Geometry: final body of the model. Coordinates: model frame, mm. Round coordinates to 2 decimals unless told otherwise and drop trailing zeros. Write each loop counter-clockwise with the first axis right and the second up, starting at its lowest first coordinate (ties: lowest second). Pieces come first, ordered by that corner, then holes. Notation, with made-up numbers: M -8,59 L 21,59 A27 cw 21,82 Z; hole C 0,-30 d11. An arc over 180 degrees is marked long. Answer as CSV lines item,"result". Start each with the question number.
Q1. Section query D-D on x = 29.5. Output: boundary loops of the cut face in (y, z) (3 decimals).
Q2. First-contact query: pin 1 (0.5 mm diameter, centred on y = -0.5, z = 0, fed in from -X); pin 2 (0.8 mm diameter, centred on y = 0, z = -15.5, fed in from -X); pin 3 (0.8 mm diameter, centred on x = 34, y = 0, fed in from +Z). Flat tips, straight axial feed; report the tip coordinate or a pass-through.
Q3. Section query B-B on x = -2.5. Output: boundary loops of the cut face in (y, z) (3 decimals).
Q4. Section query A-A on z = -2.5. Output: boundary loops of the cut face in (x, y) (3 decimals), and give its area (3 significant figures).
Q5. Ray query, probe 1 along X at (y, z) = (0.4, 4.5); probe 2 along X at (y, z) = (-0.3, 1); probe 3 along Z at (x, y) = (-8.5, 0.7). Return the intervals inside material, ascending.
Q6. Section query C-C on y = 0.3. Give the number of separate pieces and of enclosed holes in the cut face, and give its area (3 significant figures).
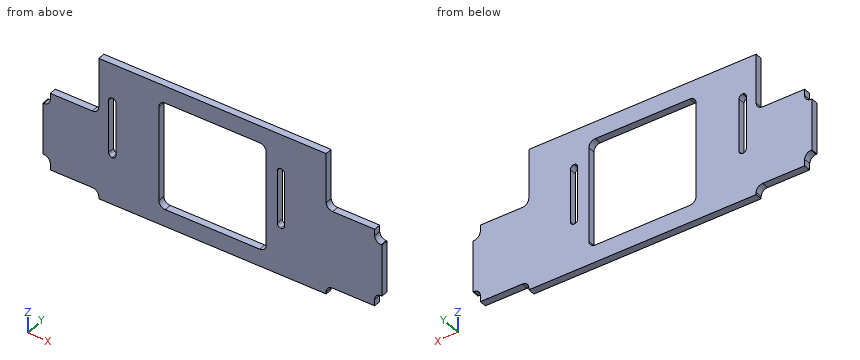
```python
from build123d import *

# Parameters (mm, degrees)
SKIZZE1_W                       = 1.7
SKIZZE1_H                       = 14
SKIZZE1_W_2                     = 25
SKIZZE1_H_2                     = 25
AUFSATZ_LINEAR_AUSTRAGEN1_DEPTH = 0.825
VERRUNDUNG1_R                   = 1.5
VERRUNDUNG2_R                   = 0.85


with BuildPart() as part:
    # Skizze1 → Aufsatz-Linear austragen1 (new, symmetric)
    # profile 1 of 3: a face of its own
    with BuildSketch(Plane(origin=(0, 0, 0), x_dir=(1, 0, 0), z_dir=(0, 1, 0))):
        Polygon((26.5, 16), (26.5, 18), (-26.5, 18), (-26.5, 16), (-26.5, -2), (-26.5, -15), (26.5, -15), (26.5, -2), align=None)
        with Locations((-23.35, 0)):
            Rectangle(SKIZZE1_W, SKIZZE1_H, mode=Mode.SUBTRACT)
        with Locations((15.95, 0)):
            Rectangle(SKIZZE1_W, SKIZZE1_H, mode=Mode.SUBTRACT)
        with Locations((0, 1.5)):
            Rectangle(SKIZZE1_W_2, SKIZZE1_H_2, mode=Mode.SUBTRACT)
    # profile 2 of 3: a face of its own
    with BuildSketch(Plane(origin=(0, 0, 0), x_dir=(1, 0, 0), z_dir=(0, 1, 0))):
        Polygon((-26.5, -2), (-26.5, 16), (-37.8, 16), (-37.8, 13), (-39.5, 13), (-39.5, 1), (-37.8, 1), (-37.8, -2), align=None)
    # profile 3 of 3: a face of its own
    with BuildSketch(Plane(origin=(0, 0, 0), x_dir=(1, 0, 0), z_dir=(0, 1, 0))):
        Polygon((37.8, 16), (26.5, 16), (26.5, -2), (37.8, -2), (37.8, 1), (39.5, 1), (39.5, 13), (37.8, 13), align=None)
    extrude(amount=AUFSATZ_LINEAR_AUSTRAGEN1_DEPTH, both=True)

    # Verrundung1
    verrundung1_edges = [part.edges().sort_by_distance(p)[0] for p in [
        (-26.5, 0, 2),
        (-37.8, 0, -1),
        (-37.8, 0, -13),
        (-26.5, 0, -16),
        (26.5, 0, -16),
        (37.8, 0, -13),
        (37.8, 0, -1),
        (26.5, 0, 2),
        (-12.5, 0, -14),
        (-12.5, 0, 11),
        (12.5, 0, 11),
        (12.5, 0, -14),
    ]]
    fillet(verrundung1_edges, radius=VERRUNDUNG1_R)

    # Verrundung2
    verrundung2_edges = [part.edges().sort_by_distance(p)[0] for p in [
        (15.1, 0, 7),
        (16.8, 0, 7),
        (15.1, 0, -7),
        (16.8, 0, -7),
        (-24.2, 0, 7),
        (-22.5, 0, 7),
        (-22.5, 0, -7),
        (-24.2, 0, -7),
    ]]
    fillet(verrundung2_edges, radius=VERRUNDUNG2_R - 0.0001)  # a hair under: the kernel refuses the full size


solid = part.part
```
Entries:
1,outline,"M -0.825,-16 L 0.825,-16 L 0.825,2 L -0.825,2 Z"
2,pin 1,"stops at x = -38"
2,pin 2,"stops at x = -37.8"
2,pin 3,"stops at z = 2"
3,outline,"M -0.825,-18 L 0.825,-18 L 0.825,-14 L -0.825,-14 Z; M -0.825,11 L 0.825,11 L 0.825,15 L -0.825,15 Z"
4,outline,"M -39.5,-0.825 L -24.2,-0.825 L -24.2,0.825 L -39.5,0.825 Z; M -22.5,-0.825 L -12.5,-0.825 L -12.5,0.825 L -22.5,0.825 Z; M 12.5,-0.825 L 15.1,-0.825 L 15.1,0.825 L 12.5,0.825 Z; M 16.8,-0.825 L 39.5,-0.825 L 39.5,0.825 L 16.8,0.825 Z"
4,area,"83.5 mm^2"
5,probe 1,"x = -26.5 to -24.2, -22.5 to -12.5, 12.5 to 15.1, 16.8 to 26.5"
5,probe 2,"x = -37.8 to -24.2, -22.5 to -12.5, 12.5 to 15.1, 16.8 to 37.8"
5,probe 3,"z = -18 to -14, 11 to 15"
6,separate pieces,"1"
6,enclosed holes,"3"
6,area,"1,530 mm^2"
